```python
from build123d import *

# Parameters (mm, degrees)
CUT_EXTRUDE1_DEPTH      = 21.178633531
CUT_EXTRUDE1_DEPTH_BACK = 21.178633531
CUT_EXTRUDE2_DEPTH      = 21.178633531
CUT_EXTRUDE2_DEPTH_BACK = 21.178633531
FILLET2_R               = 0.254
SKETCH7_R               = 0.5953125
CUT_EXTRUDE3_DEPTH      = 21.178633531


with BuildPart() as part:
    # Sketch2 → Revolve1 (revolve)
    with BuildSketch(Plane(origin=(0, 0, 0), x_dir=(0, 0, -1), z_dir=(1, 0, 0)), mode=Mode.PRIVATE) as revolve1_sk:
        with BuildLine():
            Line((-19.8628, 0), (-19.8628, 0.5953125))
            Line((-19.8628, 0.5953125), (-0.8128, 0.5953125))
            ThreePointArc((-0.8128, 0.5953125), (-0.670258675, 1.594802613), (-0.254, 2.5146))
            Line((-0.254, 2.5146), (0, 2.5146))
            Line((0, 2.5146), (0, 1.190625))
            Line((0, 1.190625), (12.7, 1.190625))
            Line((12.7, 1.190625), (12.7, 0.89296875))
            add(Edge.make_bspline(
                [(13.9192, 0), (13.9192, 2.637532552), (12.7, 0.89296875)],
                knots=[4.71238898, 4.71238898, 4.71238898, 7.005919555, 7.005919555, 7.005919555], degree=2, weights=[1, 0.411437828, 1]))
            Line((13.9192, 0), (12.7, 0))
            Line((12.7, 0), (-19.8628, 0))
        make_face()
    revolve(revolve1_sk.sketch.rotate(Axis((0, 0, 19.8628), (0, 0, -1)), 90), axis=Axis((0, 0, 19.8628), (0, 0, -1)))

    # Sketch3 → Cut-Extrude1 (cut, two sides: drawn at the far end of the back side and taken through both)
    with BuildSketch(Plane(origin=(0, 0, 0), x_dir=(1, 0, 0), z_dir=(0, 1, 0)).offset(-CUT_EXTRUDE1_DEPTH_BACK)):
        Polygon((0, -19.8628), (0.7985125, -18.822158249), (0.7985125, -20.3708), (-0.7985125, -20.3708), (-0.7985125, -18.822158249), align=None)
    extrude(amount=CUT_EXTRUDE1_DEPTH + CUT_EXTRUDE1_DEPTH_BACK, mode=Mode.SUBTRACT)

    # Sketch4 → Cut-Extrude2 (cut, two sides: drawn at the far end of the back side and taken through both)
    with BuildSketch(Plane(origin=(0, 0, 0), x_dir=(0, 0, -1), z_dir=(1, 0, 0)).offset(-CUT_EXTRUDE2_DEPTH_BACK)):
        Polygon((-20.1168, 0), (-19.0134875, 1.1033125), (-20.3708, 1.1033125), (-20.3708, -1.1033125), (-19.0134875, -1.1033125), align=None)
    extrude(amount=CUT_EXTRUDE2_DEPTH + CUT_EXTRUDE2_DEPTH_BACK, mode=Mode.SUBTRACT)

    # Fillet2
    fillet2_edges = [part.edges().sort_by_distance(p)[0] for p in [
        (-1.190625, 0, 0),
    ]]
    fillet(fillet2_edges, radius=FILLET2_R)

    # Sketch7 → Cut-Extrude3 (cut, through all)
    with BuildSketch(Plane(origin=(0, 0, 0), x_dir=(-1, 0, 0), z_dir=(0, 0, -1))):
        Circle(SKETCH7_R)
    extrude(amount=-CUT_EXTRUDE3_DEPTH, mode=Mode.SUBTRACT)


solid = part.part
```
Can you work these out from the model? Positions are in its coordinate system, mm. A direction names the side the tool comes from. Coordinates: 2 decimals unless noted, no trailing zeros. Loops run counter-clockwise (first coordinate to the right, second up) from the corner with the lowest first, then second, coordinate; pieces in that order, holes last. Notation, with made-up numbers: (71, -35) -> (86, -35) arc R24 ccw to (86, 2) -> close; hole circle Ø6 at (50, 40). An arc over 180 degrees is marked (long way). Put each result on its own line as item: value. Start each with the question number.
Q1. I want a section at A-A (z = -1). Write out the boundary of the cut face in (x, y).
Q2. If I drill on line 1 (Y direction, x = 0, z = 0.2); line 2 (Y direction, x = 0, z = 0.4); line 3 (X direction, y = -0.1, z = -9), over which ranges is the centre line in solid material (lowest first)? Write a range as [from, to].
Q3. I'm going to push flat-ended pins straight in: P1, Ø1, axis at x = 1, z = -8, coming from the +Y side; P2, Ø3, axis at x = -1.5, y = 2, coming from the +Z side; P3, Ø0.7, axis at x = 0.5, y = 0, coming from the -Z side. Where does each tip first touch, or does it pass through?
Q4. For faces 1 (the face through (0, 0, 0)), 2 (the face through (-0.26, 1.16, -6.56)), which set-ups out of +Z, -Z, +X, -X, +Y, -Y let a thin tool reach every point of the face, with its end or its side?
Taken from the geometry:
1. outline: circle Ø2.38 at (0, 0)
2. line 1: y = [-2.51, -0.6], [0.6, 2.51]
2. line 2: y = [-2.26, -0.6], [0.6, 2.26]
2. line 3: x = [-1.19, 1.19]
3. P1: stops at y = 1.08
3. P2: stops at z = 0.79
3. P3: stops at z = -13.91
4. face 1: +Z
4. face 2: -Z
